Work out the finished part from the listing and answer in its coordinate system (mm). Face numbers are marked on the shaded views. A direction names the side the tool comes from. Round coordinates to 2 decimals unless told otherwise and drop trailing zeros. Loops run counter-clockwise (first coordinate to the right, second up) from the corner with the lowest first, then second, coordinate; pieces in that order, holes last.
```python
from build123d import *

# Parameters (mm, degrees)
F0_R     = 15
F0_R_2   = 2.2
F1_DEPTH = 12
F2_T     = -1
F3_SIZE  = 2


with BuildPart() as f1:
    # F0 (on Top) → F1 (new body)
    with BuildSketch(Plane.XY):
        Circle(F0_R)
        Circle(F0_R_2, mode=Mode.SUBTRACT)
    extrude(amount=F1_DEPTH)

    # F2
    f2_openings = [f1.faces().sort_by_distance(p)[0] for p in [
        (-14.575736, 0, 12),
    ]]
    offset(amount=F2_T, openings=f2_openings)

    # F3
    f3_edges = [f1.edges().sort_by_distance(p)[0] for p in [
        (-14, 0, 1),
        (-3.2, 0, 1),
    ]]
    chamfer(f3_edges, length=F3_SIZE)


solid = f1.part
```
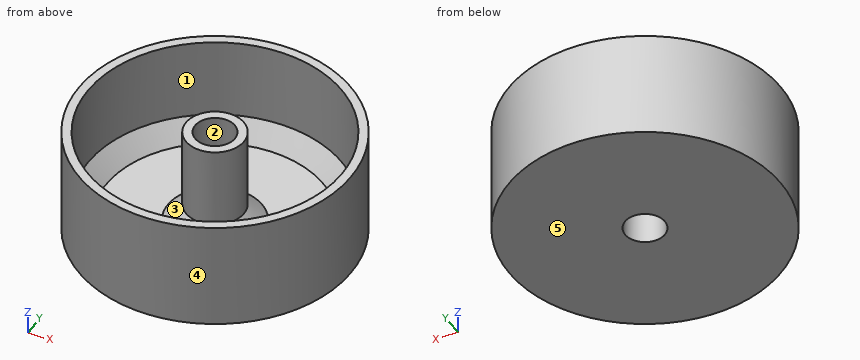
1. Find section A-A (y = 0). Write down the section's boundary in (x, z).
Answer key:
outline: (-15, 0) - (-2.2, 0) - (-2.2, 12) - (-3.2, 12) - (-3.2, 3) - (-5.2, 1) - (-12, 1) - (-14, 3) - (-14, 12) - (-15, 12) - close; (2.2, 0) - (15, 0) - (15, 12) - (14, 12) - (14, 3) - (12, 1) - (5.2, 1) - (3.2, 3) - (3.2, 12) - (2.2, 12) - close
2. Determine the mould class of the marked faces 3, 4 and 5 for opening direction Y: +Y half, -Y half, draft (parallel to the pull), parting line (faces both ways), or undercut.
Answer key:
face 3: undercut
face 4: parting line
face 5: draft
3. Find section C-C (z = 2.5). Write down the section's boundary in (x, y), then the cut area to 3 significant figures.
Answer key:
outline: circle Ø30 at (0, 0); circle Ø7.4 at (0, 0); hole circle Ø27 at (0, 0); hole circle Ø4.4 at (0, 0)
area: 162 mm2
4. Given pin 1 (1 mm diameter, centred on y = -8.5, z = 2.5, fed in from -X); pin 2 (1.5 mm diameter, centred on x = -7, z = 9.5, fed in from -Y), each flat-ended and moving along its own axis, determine where each tip first touches the part or whether it passes through.
Answer key:
pin 1: stops at x = -12.69
pin 2: stops at y = -13.64
5. Which of the six approach directions +Z, -Z, +X, -X, +Y, -Y give full straight-line access (tool end or side, diameter ignored) to the marked faces 1 and 2?
Answer key:
face 1: +Z
face 2: +Z, -Z
6. Consider probe 1 along Y at (x, z) = (0, 6.75); probe 2 along Y at (x, z) = (0.5, 6.25); probe 3 along X at (y, z) = (-1.75, 7). Determine where each line is inside the solid, lowest interval first.
Answer key:
probe 1: y = -15 to -14, -3.2 to -2.2, 2.2 to 3.2, 14 to 15
probe 2: y = -14.99 to -13.99, -3.16 to -2.14, 2.14 to 3.16, 13.99 to 14.99
probe 3: x = -14.9 to -13.89, -2.68 to -1.33, 1.33 to 2.68, 13.89 to 14.9
7. Find section D-D (z = 9). Write down the section's boundary in (x, y), then the cut area to 3 significant figures.
Answer key:
outline: circle Ø30 at (0, 0); circle Ø6.4 at (0, 0); hole circle Ø28 at (0, 0); hole circle Ø4.4 at (0, 0)
area: 108 mm2
